Build history of the part. All positions in model axes, mm. A direction names the side the tool comes from. Give positions to 0.01 mm unless a question says otherwise; leave off trailing zeros. Write each loop counter-clockwise with the first axis right and the second up, starting at its lowest first coordinate (ties: lowest second). Pieces come first, ordered by that corner, then holes. Notation, with made-up numbers: (8, 78.25) -> (60, 78.25) arc R20 ccw to (60, 89.25) -> close; hole circle Ø4 at (34, 62). An arc over 180 degrees is marked (long way). One line per question, with ' | ' between items. Start each with the question number.
(1) Drill centre lines: probe 1 along Y at (x, z) = (30, 233); probe 2 along X at (y, z) = (-19, 180); probe 3 along Y at (x, z) = (30, 31). Where is each one in solid material? Low to high. Write a range as from..to.
(2) Band-saw the part on B-B, the plane z = 180.76. Give the cut face in (x, y).
(3) Pull direction X, two halves, no side cores. Call faces 1 (the cylindrical face through (44.985, -29.34, 24.65)), 2 (the cylindrical face through (56.99, -337.15, 230.14)), 3 (the flat face through (0, -39, 176)): released by +X, released by -X, zero draft, split by the parting line, or undercut.
(4) Band-saw the part on A-A, the plane z = 21. Give the cut face in (x, y), and give its area (3 significant figures).
(5) Pin check, flat tips, straight feed: P1, Ø2, axis at x = 18, y = -231.5, coming from the -Z side; P2, Ø24, axis at x = 36, y = -33, coming from the -Z side. Stop position of each tip, or through.
(6) Tool access for faces 4 (the flat face through (30, -171, 220)), 5 (the cylindrical face through (2.85, -3.01, 123.39)), 6 (the flat face through (30, -300, 245)), 7 (the cylindrical face through (3.01, -57.15, 108.6)): list every direction of +Z, -Z, +X, -X, +Y, -Y with a clear straight run to the whole face (end or side of a thin tool).
from build123d import *

# Parameters (mm, degrees)
SKETCH1_W           = 60
SKETCH1_H           = 60
BOSS_EXTRUDE1_DEPTH = 270
SKETCH2_W           = 60
SKETCH2_H           = 50
BOSS_EXTRUDE2_DEPTH = 280
SKETCH3_R           = 15
CUT_EXTRUDE1_DEPTH  = 50
SKETCH4_R           = 27.5
CUT_EXTRUDE2_DEPTH  = 25
FILLET1_R           = 30
FILLET2_R           = 30
FILLET3_R           = 10
FILLET4_R           = 10
FILLET5_R           = 10
FILLET6_R           = 10
FILLET7_R           = 10
SKETCH5_R           = 6
CUT_EXTRUDE4_DEPTH  = 394.573373167


# Some blends are built 0.0001 mm under size
with BuildPart() as part:
    # Sketch1 → Boss-Extrude1 (new body)
    with BuildSketch(Plane.XY):
        with Locations((30, -30)):
            Rectangle(SKETCH1_W, SKETCH1_H)
    extrude(amount=BOSS_EXTRUDE1_DEPTH)

    # Sketch2 → Boss-Extrude2 (add)
    with BuildSketch(Plane.XZ.offset(60)):
        with Locations((30, 245)):
            Rectangle(SKETCH2_W, SKETCH2_H)
    extrude(amount=BOSS_EXTRUDE2_DEPTH)

    # Sketch3 → Cut-Extrude1 (cut)
    with BuildSketch(Plane(origin=(0, 0, 0), x_dir=(-1, 0, 0), z_dir=(0, 0, -1))):
        with Locations((-30, -30)):
            Circle(SKETCH3_R)
    extrude(amount=-CUT_EXTRUDE1_DEPTH, mode=Mode.SUBTRACT)

    # Sketch4 → Cut-Extrude2 (cut)
    with BuildSketch(Plane(origin=(0, 0, 220), x_dir=(-1, 0, 0), z_dir=(0, 0, -1))):
        with Locations((-30, -300)):
            Circle(SKETCH4_R)
    extrude(amount=-CUT_EXTRUDE2_DEPTH, mode=Mode.SUBTRACT)

    # Fillet1
    fillet1_edges = [part.edges().sort_by_distance(p)[0] for p in [
        (60, -170, 270),
    ]]
    fillet(fillet1_edges, radius=FILLET1_R)

    # Fillet2
    fillet2_edges = [part.edges().sort_by_distance(p)[0] for p in [
        (0, -170, 270),
    ]]
    fillet(fillet2_edges, radius=FILLET2_R - 0.0001)  # a hair under: the kernel refuses the full size

    # Fillet3
    fillet3_edges = [part.edges().sort_by_distance(p)[0] for p in [
        (60, 0, 120),
        (51.213203436, 0, 261.213203436),
        (0, 0, 120.00005),
        (8.786767275, 0, 261.213232725),
    ]]
    fillet(fillet3_edges, radius=FILLET3_R)

    # Fillet4
    fillet4_edges = [part.edges().sort_by_distance(p)[0] for p in [
        (60, -35, 0),
        (30, 0, 0),
        (0, -35, 0),
        (2.928932188, -2.928932188, 0),
        (57.071067812, -2.928932188, 0),
    ]]
    fillet(fillet4_edges, radius=FILLET4_R)

    # Fillet5
    fillet5_edges = [part.edges().sort_by_distance(p)[0] for p in [
        (60, -60, 115),
        (0, -60, 115),
        (30, -60, 0),
        (2.928932188, -60, 2.928932188),
        (57.071067812, -60, 2.928932188),
    ]]
    fillet(fillet5_edges, radius=FILLET5_R)

    # Fillet6
    # the kernel refuses this fillet: 10 mm, written as the material it adds along each edge
    with BuildSketch(Plane(origin=(50, -60, 220), x_dir=(0, 0, -1), z_dir=(-1, 0, 0))) as fillet6_piece_1:
        with BuildLine():
            CenterArc((FILLET6_R, FILLET6_R), FILLET6_R, 180, 90)
            Line((0, FILLET6_R), (0, 0))
            Line((0, 0), (FILLET6_R, 0))
        make_face()
    extrude(amount=40)
    with BuildSketch(Plane(origin=(50, -50, 220), x_dir=(-0.8017442392976486, 0.5976672776328272, 0), z_dir=(-0.5976672776328272, -0.8017442392976486, 0))) as fillet6_piece_2_section:
        with BuildLine():
            CenterArc((10 + FILLET6_R, FILLET6_R), FILLET6_R, 180, 90)
            Line((10 + FILLET6_R, 0), (10, 0))
            Line((10, 0), (10, FILLET6_R))
        make_face()
    fillet6_piece_2 = revolve(axis=Axis((50, -50, 220), (0, 0, -1)), revolution_arc=233.296989237, mode=Mode.PRIVATE)
    fillet6_piece_2 = split(fillet6_piece_2, bisect_by=Plane(origin=(60, -57.499389328, 216.883716878), z_dir=(-1, 0, 0)), keep=Keep.TOP, mode=Mode.PRIVATE)
    add(fillet6_piece_2)
    with BuildSketch(Plane(origin=(10, -50, 220), x_dir=(0.8017442392976489, 0.5976672776328267, 0), z_dir=(0.5976672776328267, -0.8017442392976489, 0))) as fillet6_piece_3_section:
        with BuildLine():
            CenterArc((10 + FILLET6_R, -FILLET6_R), FILLET6_R, 90, 90)
            Line((10, -FILLET6_R), (10, 0))
            Line((10, 0), (10 + FILLET6_R, 0))
        make_face()
    fillet6_piece_3 = revolve(axis=Axis((10, -50, 220), (0, 0, 1)), revolution_arc=233.296989237, mode=Mode.PRIVATE)
    fillet6_piece_3 = split(fillet6_piece_3, bisect_by=Plane(origin=(0, -57.499389357, 216.883716675), z_dir=(1, 0, 0)), keep=Keep.TOP, mode=Mode.PRIVATE)
    add(fillet6_piece_3)

    # Fillet7
    fillet7_edges = [part.edges().sort_by_distance(p)[0] for p in [
        (60, -340, 230),
        (51.213203436, -340, 261.213203436),
        (0, -340, 230.00005),
        (8.786767275, -340, 261.213232725),
    ]]
    fillet(fillet7_edges, radius=FILLET7_R)

    # Sketch5 → Cut-Extrude4 (cut, through all)
    with BuildSketch(Plane.XZ.offset(60)):
        with Locations((30, 180.76)):
            Circle(SKETCH5_R)
    extrude(amount=-CUT_EXTRUDE4_DEPTH, mode=Mode.SUBTRACT)


solid = part.part
Results:
1) probe 1: y = -340..-327.5, -272.5..0 | probe 2: x = 0..24.05, 35.95..60 | probe 3: y = -60..-45, -15..0
2) outline: (0, -50) arc R10 ccw to (10, -60) -> (24, -60) -> (24, 0) -> (10, 0) arc R10 ccw to (0, -10) -> close; (36, -60) -> (50, -60) arc R10 ccw to (60, -50) -> (60, -10) arc R10 ccw to (50, 0) -> (36, 0) -> close
3) face 1: undercut | face 2: released by +X | face 3: released by -X
4) outline: (0, -50) arc R10 ccw to (10, -60) -> (50, -60) arc R10 ccw to (60, -50) -> (60, -10) arc R10 ccw to (50, 0) -> (10, 0) arc R10 ccw to (0, -10) -> close; hole circle Ø30 at (30, -30) | area: 2,810 mm²
5) P1: stops at z = 220 | P2: stops at z = 0
6) face 4: -Z, +X, -X, -Y | face 5: +Z, -Z, -X, +Y | face 6: -Z | face 7: -Z, -X, -Y
